Read the model definition and answer for the solid it produces. Units are mm, in the model's axes. Coordinates: 2 decimals unless noted, no trailing zeros. Write each loop counter-clockwise with the first axis right and the second up, starting at its lowest first coordinate (ties: lowest second). Pieces come first, ordered by that corner, then holes.
1) The part is cut by section C-C (z = 42). Determine the outline of the cut face in (x, y), then the cut area to 3 significant figures.
2) Each of these flat-tipped pins is pushed along its axis until it touches: pin 1 Ø1.2 at (x, y) = (-1.5, 1.5) entering from +Z; pin 2 Ø0.8 at (x, y) = (-46, 3) entering from -Z; pin 3 Ø7 at (x, z) = (-65, 5) entering from +Y; pin 4 Ø1.2 at (y, z) = (2, 51) entering from +X. Where does it stop, or does it pass through?
3) The part is cut by section B-B (z = 5). Determine the outline of the cut face in (x, y).
4) The part is cut by section A-A (x = -65). Determine the outline of the cut face in (y, z).
5) Find the intervals of material crossed by line 1 (Z direction, x = 46, y = 2.7); line 2 (X direction, y = 0.45, z = 44); line 3 (X direction, y = 3.6, z = -4), in increasing order.
6) The part is cut by section D-D (x = 70). Determine the outline of the cut face in (y, z).
from build123d import *

# Parameters (mm, degrees)
BOSS_EXTRUDE1_DEPTH = 4
SKETCH2_R           = 4
SKETCH2_R_2         = 3.5
SKETCH2_R_3         = 2.5
SKETCH2_W           = 13
SKETCH2_H           = 19.5
CUT_EXTRUDE1_DEPTH  = 5
CUT_EXTRUDE2_DEPTH  = 6


with BuildPart() as part:
    # Sketch1 → Boss-Extrude1 (new body)
    with BuildSketch(Plane(origin=(0, 0, 0), x_dir=(1, 0, 0), z_dir=(0, 1, 0))):
        Polygon((-55, -50), (-43, -50), (-43, -54), (-23, -54), (-23, -50), (23, -50), (23, -54), (43, -54), (43, -50), (55, -50), (55, -54), (75, -54), (75, -50), (100, -50), (100, 50), (75, 50), (75, 54), (55, 54), (55, 50), (43, 50), (43, 54), (23, 54), (23, 50), (-23, 50), (-23, 54), (-43, 54), (-43, 50), (-55, 50), (-55, 54), (-75, 54), (-75, 50), (-100, 50), (-100, -50), (-75, -50), (-75, -54), (-55, -54), align=None)
    extrude(amount=BOSS_EXTRUDE1_DEPTH)

    # Sketch2 → Cut-Extrude1 (cut, through all)
    with BuildSketch(Plane.XZ):
        with Locations((-65, 5)):
            Circle(SKETCH2_R)
        with Locations((26, 5)):
            Circle(SKETCH2_R_2)
        with Locations((46, 5)):
            Circle(SKETCH2_R_3)
        with Locations((58, 5)):
            Circle(SKETCH2_R_3)
        with Locations((70, 5)):
            Circle(SKETCH2_R_3)
        with Locations((-40, 5)):
            Rectangle(SKETCH2_W, SKETCH2_H)
    extrude(amount=-CUT_EXTRUDE1_DEPTH, mode=Mode.SUBTRACT)

    # Sketch3 → Cut-Extrude2 (cut)
    with BuildSketch(Plane.XZ):
        Polygon((-51.1, -50), (-46.9, -50), (-46.9, -40), (-44.5, -40), (-44.5, -39), (-45.25, -39), (-45.25, -36.5), (-46.9, -36.5), (-46.9, -33), (-51.1, -33), (-51.1, -36.5), (-52.75, -36.5), (-52.75, -39), (-53.5, -39), (-53.5, -40), (-51.1, -40), align=None)
        Polygon((46.9, -50), (46.9, -40), (44.5, -40), (44.5, -39), (45.25, -39), (45.25, -36.5), (46.9, -36.5), (46.9, -33), (51.1, -33), (51.1, -36.5), (52.75, -36.5), (52.75, -39), (53.5, -39), (53.5, -40), (51.1, -40), (51.1, -50), align=None)
    cut_extrude2 = extrude(amount=-CUT_EXTRUDE2_DEPTH, mode=Mode.SUBTRACT)

    # Mirror1: Cut-Extrude2 across plane
    add(cut_extrude2.mirror(Plane.XY), mode=Mode.SUBTRACT)


solid = part.part
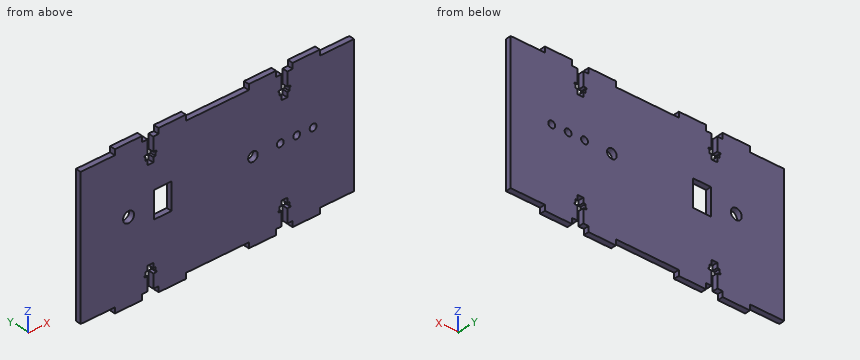
Reported:
1. outline: (-100, 0) - (-51.1, 0) - (-51.1, 4) - (-100, 4) - close; (-46.9, 0) - (46.9, 0) - (46.9, 4) - (-46.9, 4) - close; (51.1, 0) - (100, 0) - (100, 4) - (51.1, 4) - close
1. area: 766 mm2
2. pin 1: stops at z = 50
2. pin 2: stops at z = -50
2. pin 3: passes through
2. pin 4: stops at x = 75
3. outline: (-100, 0) - (-69, 0) - (-69, 4) - (-100, 4) - close; (-61, 0) - (-46.5, 0) - (-46.5, 4) - (-61, 4) - close; (-33.5, 0) - (22.5, 0) - (22.5, 4) - (-33.5, 4) - close; (29.5, 0) - (43.5, 0) - (43.5, 4) - (29.5, 4) - close; (48.5, 0) - (55.5, 0) - (55.5, 4) - (48.5, 4) - close; (60.5, 0) - (67.5, 0) - (67.5, 4) - (60.5, 4) - close; (72.5, 0) - (100, 0) - (100, 4) - (72.5, 4) - close
4. outline: (0, -54) - (4, -54) - (4, 1) - (0, 1) - close; (0, 9) - (4, 9) - (4, 54) - (0, 54) - close
5. line 1: z = -50 to -40, -36.5 to 2.5, 7.5 to 36.5, 40 to 50
5. line 2: x = -100 to -51.1, -46.9 to 46.9, 51.1 to 100
5. line 3: x = -100 to -46.5, -33.5 to 100
6. outline: (0, -54) - (4, -54) - (4, 2.5) - (0, 2.5) - close; (0, 7.5) - (4, 7.5) - (4, 54) - (0, 54) - close
